Could you check a few things on this model? Use its own coordinates, in mm. Coordinates: 2 decimals unless noted, no trailing zeros. Write each loop counter-clockwise with the first axis right and the second up, starting at its lowest first coordinate (ties: lowest second). Pieces come first, ordered by that corner, then holes. Notation, with made-up numbers: M 76.5,-33.5 L 107.5,-33.5 A22 ccw 107.5,4.5 Z; hole C 3.5,83 d1. An arc over 180 degrees is marked long. Write item = value, one per line.
```python
from build123d import *

# Parameters (mm, degrees)
KES_EKSTR_ZYON2_DEPTH = 10
IZIM4_R               = 0.5
IZIM6_R               = 0.5


with BuildPart() as part:
    # Çizim1 → Döndür2 (revolve)
    with BuildSketch(Plane.XY, mode=Mode.PRIVATE) as d_nd_r2_sk:
        with BuildLine():
            Line((0, 0), (10, 0))
            Line((10, 0), (10, 4.346574423))
            Line((10, 4.346574423), (9, 4.346574423))
            Line((9, 4.346574423), (9, 20))
            ThreePointArc((9, 20), (7.535533906, 23.535533906), (4, 25))
            Line((4, 25), (0, 25))
            Line((0, 25), (0, 0))
        make_face()
    revolve(d_nd_r2_sk.sketch.rotate(Axis((0, 25, 0), (0, -1, 0)), 180), axis=Axis((0, 25, 0), (0, -1, 0)))

    # Çizim2 → Kes-Ekstrüzyon2 (cut)
    with BuildSketch(Plane.XZ):
        Polygon((-6.667667497, 7.452664634), (1.504038202, 9.886246461), (0.616082269, 11.592722448), (-7.506944277, 10), align=None)
    extrude(amount=-KES_EKSTR_ZYON2_DEPTH, mode=Mode.SUBTRACT)

    # Süpür1: sweep along a curve in space
    with BuildLine() as s_p_r1_path:
        Line((-1.443878782, 1.853325266, 5.182498136), (-1.443878782, -29.967465354, 5.182498136))
    # Çizim4 → Süpür1 (sweep)
    with BuildSketch(Plane(origin=(-1.443878782, -29.967465354, 5.182498136), x_dir=(-1, 0, 0), z_dir=(0, -1, 0))):
        Circle(IZIM4_R)
    sweep(path=s_p_r1_path.line)

    # Süpür2: sweep along a curve in space
    with BuildLine() as s_p_r2_path:
        Line((1.793792857, 0, -4.435841685), (1.793792857, -42.508039012, -4.435841685))
    # Çizim6 → Süpür2 (sweep)
    with BuildSketch(Plane(origin=(1.793792857, -42.508039012, -4.435841685), x_dir=(-1, 0, 0), z_dir=(0, -1, 0))):
        Circle(IZIM6_R)
    sweep(path=s_p_r2_path.line)


solid = part.part
```
Item 1: Imagine slicing it at C-C (y = -37). Write out the boundary of the cut face in (x, z), and give its area (3 significant figures).
Numbers:
outline = C 1.79,-4.44 d1
area = 0.785 mm²
Item 2: If I drill on line 1 along Y through (x, z) = (-7, -6); line 2 along Y through (x, z) = (-2.25, -1.75); line 3 along X through (y, z) = (3.5, 1.25), over which ranges is the centre line in solid material (lowest first)?
Numbers:
line_1 = 0 to 4.35
line_2 = 0 to 25
line_3 = -9.92 to 9.92
Item 3: If we mould it in two halves opening along X, with no side actions, what happens to faces 1 (the face through (-2.639, 2.143, 8.652)), 2 (the face through (6.633, 12.283, -6.083)), 3 (the face through (7, 4.347, -6))? For each: pulls with the +X half, pulls with the -X half, needs draft (parallel to the pull), parting line crosses it, or undercut.
Numbers:
face_1 = pulls with the -X half
face_2 = parting line crosses it
face_3 = needs draft
Item 4: Imagine slicing it at A-A (y = 8). Write out the boundary of the cut face in (x, z), and give its area (3 significant figures).
Numbers:
outline = C 0,0 d18
area = 254 mm²
Item 5: I'm going to push flat-ended pins straight in: P1, Ø5, axis at x = -3, y = -29, coming from the +Z side; P2, Ø6, axis at y = 8, z = -3.5, coming from the -X side; P3, Ø1, axis at x = 0, y = -17, coming from the -Z side; P4, Ø2, axis at x = 4, z = 0.5, coming from the -Y side. Where does each tip first touch, or does it pass through?
Numbers:
P1 = 5.68
P2 = -8.99
P3 = through
P4 = 0
Item 6: Imagine slicing it at B-B (y = -9). Write out the boundary of the cut face in (x, z).
Numbers:
outline = C -1.44,5.18 d1; C 1.79,-4.44 d1
